```python
from build123d import *

# Parameters (mm, degrees)
PAD_DEPTH       = 9
POCKET_DEPTH    = 5
POCKET001_DEPTH = 20
SKETCH003_R     = 1.5
PAD001_DEPTH    = 3.5


with BuildPart() as part:
    # Sketch → Pad (new body)
    with BuildSketch(Plane.XY):
        with BuildLine():
            Line((-11.5, 17.5), (11.5, 17.5))
            ThreePointArc((14, 15), (13.267767, 16.767767), (11.5, 17.5))
            Line((14, 15), (14, -15))
            ThreePointArc((11.5, -17.5), (13.267767, -16.767767), (14, -15))
            Line((11.5, -17.5), (-11.5, -17.5))
            ThreePointArc((-14, -15), (-13.267767, -16.767767), (-11.5, -17.5))
            Line((-14, -15), (-14, 15))
            ThreePointArc((-11.5, 17.5), (-13.267767, 16.767767), (-14, 15))
        make_face()
    extrude(amount=PAD_DEPTH)

    # Sketch001 (on Face10 of Pad) → Pocket (cut)
    with BuildSketch(Plane.XY.offset(9)):
        with BuildLine():
            Line((-11, 15.5), (11, 15.5))
            ThreePointArc((12, 14.5), (11.707107, 15.207107), (11, 15.5))
            Line((12, 14.5), (12, -8.5))
            Line((12, -8.5), (10.5, -9.76))
            Line((10.5, -9.76), (10.5, -11.79))
            Line((10.5, -11.79), (12, -13.05))
            Line((12, -13.05), (12, -18.05))
            Line((-12, -18.05), (12, -18.05))
            Line((-12, -13.05), (-12, -18.05))
            Line((-10.5, -11.79), (-12, -13.05))
            Line((-10.5, -9.76), (-10.5, -11.79))
            Line((-12, -8.5), (-10.5, -9.76))
            Line((-12, 14.5), (-12, -8.5))
            ThreePointArc((-11, 15.5), (-11.707107, 15.207107), (-12, 14.5))
        make_face()
    extrude(amount=-POCKET_DEPTH, mode=Mode.SUBTRACT)

    # Sketch002 (on Face9 of Pocket) → Pocket001 (cut)
    with BuildSketch(Plane(origin=(0, 17.5, 0), x_dir=(-1, 0, 0), z_dir=(0, 0.984808, -0.173648))):
        with BuildLine():
            ThreePointArc((-1.5, 3.16327), (0, 1.66327), (1.5, 3.16327))
            Line((1.5, 8.86327), (1.5, 3.16327))
            Line((-1.5, 8.86327), (1.5, 8.86327))
            Line((-1.5, 8.86327), (-1.5, 3.16327))
        make_face()
    extrude(amount=-POCKET001_DEPTH, mode=Mode.SUBTRACT)

    # Sketch003 (on Face4 of Pocket001) → Pad001 (join)
    with BuildSketch(Plane(origin=(0, 0, 0), x_dir=(1, 0, 0), z_dir=(0, 0, -1))):
        with BuildLine():
            ThreePointArc((-20, 11), (-26, 5), (-20, -1))
            Line((-20, -1), (20, -1))
            ThreePointArc((20, -1), (26, 5), (20, 11))
            Line((-20, 11), (20, 11))
        make_face()
        with Locations((-20, 5)):
            Circle(SKETCH003_R, mode=Mode.SUBTRACT)
        with Locations((20, 5)):
            Circle(SKETCH003_R, mode=Mode.SUBTRACT)
    extrude(amount=-PAD001_DEPTH)


solid = part.part
```
Geometry: final body of the model. Coordinates: model frame, mm. A direction names the side the tool comes from. Coordinates: 2 decimals unless noted, no trailing zeros. Order: outer loops, then holes, each group sorted by start corner. A loop starts at its lowest first (then second) coordinate and runs counter-clockwise, first axis right, second up. Notation, with made-up numbers: M -6,42 L 13,42 A16 cw 13,54 Z; hole C 78.5,-7 d8. An arc over 180 degrees is marked long. Answer as CSV lines item,"result".
Q1. Set-up query: faces 4 (the flat face through (11.24, -12.41, 6.54)), 5 (the cylindrical face through (26, -5, 2)), 6 (the flat face through (-18.8, -3.8, 3.5)), 7 (the flat face through (0, 0, 0)), 8 (the flat face through (-17, 1, 2)). Return all of +Z, -Z, +X, -X, +Y, -Y with unobstructed straight access to the full face (end or side cutting, diameter ignored); none if empty.
Answers:
face 4,"+Z, -Y"
face 5,"+Z, -Z, +X"
face 6,"+Z, -X, +Y, -Y"
face 7,"-Z, +X, -X, +Y, -Y"
face 8,"+Z, -Z, -X, +Y"
Q2. First-contact query: P1, Ø1, axis at y = -11, z = 7.5, coming from the +X side; P2, Ø2.5, axis at x = -20, y = -5, coming from the -Z side; P3, Ø6, axis at x = 18.5, y = -5, coming from the +Z side; P4, Ø12, axis at x = -3, y = 3, coming from the +Z side. Flat tips, straight axial feed; report the tip coordinate or a pass-through.
Answers:
P1,"stops at x = 14"
P2,"passes through"
P3,"stops at z = 3.5"
P4,"stops at z = 4"
Q3. Section B-B on y = -5. Return the cut outline in (x, z), and give its area (3 significant figures).
Answers:
outline,"M -26,0 L -21.5,0 L -21.5,3.5 L -26,3.5 Z; M -18.5,0 L 18.5,0 L 18.5,3.5 L 14,3.5 L 14,9 L 12,9 L 12,4 L -12,4 L -12,9 L -14,9 L -14,3.5 L -18.5,3.5 Z; M 21.5,0 L 26,0 L 26,3.5 L 21.5,3.5 Z"
area,"195 mm^2"
Q4. Section D-D on x = 16. Return the cut outline in (y, z).
Answers:
outline,"M -11,0 L 1,0 L 1,3.5 L -11,3.5 Z"
Q5. Section A-A on z = 5.75. Return the cut outline in (x, y), and give its area (3 significant figures).
Answers:
outline,"M -14,-15 A2.5 ccw -12,-17.45 L -12,-13.05 L -10.5,-11.79 L -10.5,-9.76 L -12,-8.5 L -12,14.5 A1 cw -11,15.5 L -1.5,15.5 L -1.5,17.5 L -11.5,17.5 A2.5 ccw -14,15 Z; M 1.5,15.5 L 11,15.5 A1 cw 12,14.5 L 12,-8.5 L 10.5,-9.76 L 10.5,-11.79 L 12,-13.05 L 12,-17.45 A2.5 ccw 14,-15 L 14,15 A2.5 ccw 11.5,17.5 L 1.5,17.5 Z"
area,"187 mm^2"
Q6. Draft query along Y for faces 1 (the cylindrical face through (-11.699, 15.215, 6.535)), 2 (the cylindrical face through (-26, -5, 2)), 3 (the cylindrical face through (-13, 17, 4)). Return one class per face: pulls with the +Y half, pulls with the -Y half, needs draft (parallel to the pull), parting line crosses it, or undercut.
Answers:
face 1,"undercut"
face 2,"parting line crosses it"
face 3,"pulls with the +Y half"
Q7. Section C-C on y = 3.5. Return the cut outline in (x, z), and give its area (3 significant figures).
Answers:
outline,"M -14,0 L 14,0 L 14,9 L 12,9 L 12,4 L -12,4 L -12,9 L -14,9 Z"
area,"132 mm^2"
Q8. Line query: probe 1 along X at (y, z) = (-5, 1); probe 2 along Y at (x, z) = (-20, 2.75); probe 3 along X at (y, z) = (0, 8). Output: solid intervals per line, ascending. Write a range as [from, to].
Answers:
probe 1,"x = [-26, -21.5], [-18.5, 18.5], [21.5, 26]"
probe 2,"y = [-11, -6.5], [-3.5, 1]"
probe 3,"x = [-14, -12], [12, 14]"
